Could you check a few things on this drawing? It's one solid part, dimensions in mm from its lowest x, y, z. Round coordinates to 2 decimals unless told otherwise and drop trailing zeros. Loops run counter-clockwise (first coordinate to the right, second up) from the corner with the lowest first, then second, coordinate; pieces in that order, holes last. Notation, with made-up numbers: (-1, -4.75) -> (58, -4.75) arc R23 cw to (58, 3.25) -> close; hole circle Ø10 at (86, 27). An arc over 180 degrees is marked (long way). Put each result on its own line as item: value. Start each with the question number.
1. Imagine slicing it at D-D, the plane z = 12.7. Please give me the cut outline in (x, y) (1 decimal).
2. Imagine slicing it at B-B, the plane z = 38.1. Please give me the cut outline in (x, y) (1 decimal).
3. Imagine slicing it at C-C, the plane x = 12.7. Please give me the cut outline in (y, z) (1 decimal).
4. I need wall thicknesses on line 1 (Z direction, x = 38.1, y = 1.6); line 2 (Z direction, x = 12.7, y = 1.4); line 3 (X direction, y = 1.5, z = 45). Which ranges of each line are inside material? Lowest first, please. Write a range as [from, to].
5. Imagine slicing it at A-A, the plane x = 38.1. Please give me the cut outline in (y, z) (1 decimal), and give its area (3 significant figures).
6. I'm going to push flat-ended pins straight in: P1, Ø1, axis at x = 9, y = 1, coming from the +Z side; P2, Ø8.5, axis at x = 25.4, z = 12.7, coming from the +Y side (3 decimals); P3, Ø1.6, axis at y = 1.5, z = 33.5, coming from the -X side; P4, Ø4, axis at x = 38.1, z = 12.7, coming from the +Y side. Where does each tip first touch, or does it pass through?
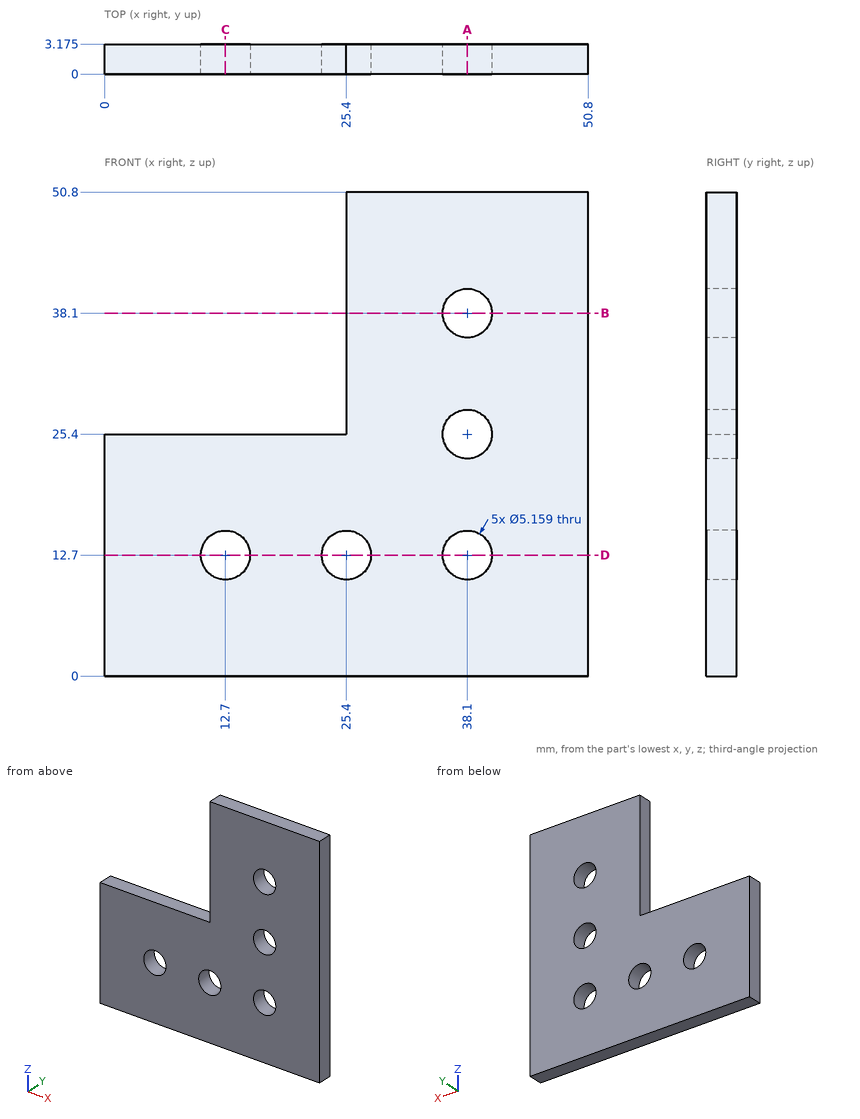
Entries:
1. outline: (0, 0) -> (10.1, 0) -> (10.1, 3.2) -> (0, 3.2) -> close; (15.3, 0) -> (22.8, 0) -> (22.8, 3.2) -> (15.3, 3.2) -> close; (28, 0) -> (35.5, 0) -> (35.5, 3.2) -> (28, 3.2) -> close; (40.7, 0) -> (50.8, 0) -> (50.8, 3.2) -> (40.7, 3.2) -> close
2. outline: (25.4, 0) -> (35.5, 0) -> (35.5, 3.2) -> (25.4, 3.2) -> close; (40.7, 0) -> (50.8, 0) -> (50.8, 3.2) -> (40.7, 3.2) -> close
3. outline: (0, 0) -> (3.2, 0) -> (3.2, 10.1) -> (0, 10.1) -> close; (0, 15.3) -> (3.2, 15.3) -> (3.2, 25.4) -> (0, 25.4) -> close
4. line 1: [0, 10.12], [15.28, 22.82], [27.98, 35.52], [40.68, 50.8]
4. line 2: [0, 10.12], [15.28, 25.4]
4. line 3: [25.4, 50.8]
5. outline: (0, 0) -> (3.2, 0) -> (3.2, 10.1) -> (0, 10.1) -> close; (0, 15.3) -> (3.2, 15.3) -> (3.2, 22.8) -> (0, 22.8) -> close; (0, 28) -> (3.2, 28) -> (3.2, 35.5) -> (0, 35.5) -> close; (0, 40.7) -> (3.2, 40.7) -> (3.2, 50.8) -> (0, 50.8) -> close
5. area: 112 mm^2
6. P1: z = 25.4
6. P2: y = 3.175
6. P3: x = 25.4
6. P4: through
